For this review, take the finished solid that the model builds, in its own axes (mm). Round coordinates to 2 decimals unless told otherwise and drop trailing zeros. Order: outer loops, then holes, each group sorted by start corner. A loop starts at its lowest first (then second) coordinate and runs counter-clockwise, first axis right, second up. Notation, with made-up numbers: (-34.5, 44) - (-2.5, 44) arc R9 cw to (-2.5, 50) - close; hole circle Ø5 at (-12.5, 11). An arc over 180 degrees is marked (long way). One line per item, written item: value.
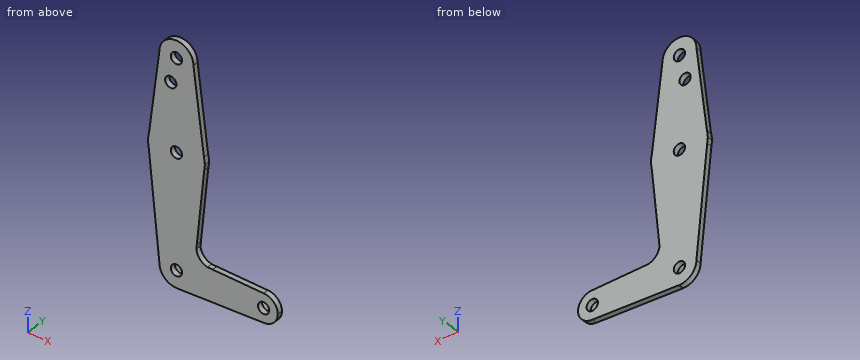
```python
from build123d import *

# Parameters (mm, degrees)
F0_R     = 3.175
F1_DEPTH = 3.048


with BuildPart() as f1:
    # F0 (on Front) → F1 (new body)
    with BuildSketch(Plane.XZ):
        with BuildLine():
            ThreePointArc((-9.525, 66.5221907973), (0, 56.9971907973), (9.525, 66.5221907973))
            ThreePointArc((9.525, 66.5221907973), (0, 76.0471907973), (-9.525, 66.5221907973))
        make_face()
        with Locations((0, 66.5221907973)):
            Circle(F0_R, mode=Mode.SUBTRACT)
        with BuildLine():
            Line((15.3865384615, 19.629883105), (9.525, 66.5221907973))
            ThreePointArc((9.525, 66.5221907973), (0, 56.9971907973), (-9.525, 66.5221907973))
            Line((-9.525, 66.5221907973), (-15.3865384615, 19.629883105))
            ThreePointArc((-15.3865384615, 19.629883105), (0, 31.5971907973), (15.3865384615, 19.629883105))
        make_face()
        with Locations((-3.175, 52.341658622)):
            Circle(F0_R, mode=Mode.SUBTRACT)
        with BuildLine():
            Line((15.875, 15.7221907973), (15.3865384615, 19.629883105))
            ThreePointArc((15.3865384615, 19.629883105), (0, 31.5971907973), (-15.3865384615, 19.629883105))
            Line((-15.3865384615, 19.629883105), (-15.875, 15.7221907973))
            Line((-15.875, 15.7221907973), (-15.5606435644, 12.5786264409))
            ThreePointArc((-15.5606435644, 12.5786264409), (0, -0.1528092027), (15.5606435644, 12.5786264409))
            Line((15.5606435644, 12.5786264409), (15.875, 15.7221907973))
        make_face()
        with Locations((0, 15.7221907973)):
            Circle(F0_R, mode=Mode.SUBTRACT)
        with BuildLine():
            ThreePointArc((15.875, 15.7221907973), (15.7524112928, 17.6912422089), (15.3865384615, 19.629883105))
            Line((15.3865384615, 19.629883105), (15.875, 15.7221907973))
        make_face()
        with BuildLine():
            Line((-15.875, 15.7221907973), (-15.3865384615, 19.629883105))
            ThreePointArc((-15.3865384615, 19.629883105), (-15.7524112928, 17.6912422089), (-15.875, 15.7221907973))
        make_face()
        with BuildLine():
            ThreePointArc((15.5606435644, 12.5786264409), (15.7962153946, 14.1425692579), (15.875, 15.7221907973))
            Line((15.875, 15.7221907973), (15.5606435644, 12.5786264409))
        make_face()
        with BuildLine():
            Line((-15.5606435644, 12.5786264409), (-15.875, 15.7221907973))
            ThreePointArc((-15.875, 15.7221907973), (-15.7962153946, 14.1425692579), (-15.5606435644, 12.5786264409))
        make_face()
        with BuildLine():
            Line((11.4104326497, -28.9234827055), (15.5606435644, 12.5786264409))
            ThreePointArc((15.5606435644, 12.5786264409), (0, -0.1528092027), (-15.5606435644, 12.5786264409))
            Line((-15.5606435644, 12.5786264409), (-9.525, -47.7778092027))
            ThreePointArc((-9.525, -47.7778092027), (-6.7351920908, -41.0426171119), (0, -38.2528092027))
            ThreePointArc((0, -38.2528092027), (0.309842749, -38.2578500394), (0.6193575471, -38.272967214))
            Line((0.6193575471, -38.272967214), (10.4435098772, -38.5927104307))
            Line((10.4435098772, -38.5927104307), (11.1406480746, -31.6213284562))
            ThreePointArc((11.1406480746, -31.6213284562), (11.1596842937, -30.260819974), (11.4104326497, -28.9234827055))
        make_face()
        with BuildLine():
            Line((11.1406480746, -31.6213284562), (11.4104326497, -28.9234827055))
            ThreePointArc((11.4104326497, -28.9234827055), (11.1596842937, -30.260819974), (11.1406480746, -31.6213284562))
        make_face()
        with BuildLine():
            ThreePointArc((0, -38.2528092027), (-6.7351920908, -41.0426171119), (-9.525, -47.7778092027))
            ThreePointArc((-9.525, -47.7778092027), (-6.7351920908, -54.5130012935), (0, -57.3028092027))
            Line((0, -57.3028092027), (0.6193575471, -57.2826511913))
            ThreePointArc((0.6193575471, -57.2826511913), (6.9507195899, -54.2903449747), (9.525, -47.7778092027))
            ThreePointArc((9.525, -47.7778092027), (6.9507195899, -41.2652734306), (0.6193575471, -38.272967214))
            Line((0.6193575471, -38.272967214), (0, -38.2528092027))
        make_face()
        with Locations((0, -47.7778092027)):
            Circle(F0_R, mode=Mode.SUBTRACT)
        with BuildLine():
            ThreePointArc((17.370144363, -38.8181491572), (13.0593477477, -36.2550264457), (11.1406480746, -31.6213284562))
            Line((11.1406480746, -31.6213284562), (10.4435098772, -38.5927104307))
            Line((10.4435098772, -38.5927104307), (17.370144363, -38.8181491572))
        make_face()
        with BuildLine():
            Line((0.6193575471, -57.2826511913), (0, -57.3028092027))
            ThreePointArc((0, -57.3028092027), (0.309842749, -57.297768366), (0.6193575471, -57.2826511913))
        make_face()
        with BuildLine():
            Line((17.370144363, -38.8181491572), (10.4435098772, -38.5927104307))
            Line((10.4435098772, -38.5927104307), (9.525, -47.7778092027))
            ThreePointArc((9.525, -47.7778092027), (6.9507195899, -54.2903449747), (0.6193575471, -57.2826511913))
            Line((0.6193575471, -57.2826511913), (48.7761460245, -55.7153092027))
            ThreePointArc((48.7761460245, -55.7153092027), (40.8386460245, -47.7778092027), (48.7761460245, -39.8403092027))
            Line((48.7761460245, -39.8403092027), (20.2621190411, -38.9122732358))
            ThreePointArc((20.2621190411, -38.9122732358), (18.8118135488, -38.9978870226), (17.370144363, -38.8181491572))
        make_face()
        with BuildLine():
            Line((20.2621190411, -38.9122732358), (17.370144363, -38.8181491572))
            ThreePointArc((17.370144363, -38.8181491572), (18.8118135488, -38.9978870226), (20.2621190411, -38.9122732358))
        make_face()
        with BuildLine():
            ThreePointArc((48.7761460245, -39.8403092027), (40.8386460245, -47.7778092027), (48.7761460245, -55.7153092027))
            ThreePointArc((48.7761460245, -55.7153092027), (54.3888061001, -53.3904692783), (56.7136460245, -47.7778092027))
            ThreePointArc((56.7136460245, -47.7778092027), (54.3888061001, -42.165149127), (48.7761460245, -39.8403092027))
        make_face()
        with Locations((48.7761460245, -47.7778092027)):
            Circle(F0_R, mode=Mode.SUBTRACT)
        with BuildLine():
            Line((9.525, -47.7778092027), (10.4435098772, -38.5927104307))
            Line((10.4435098772, -38.5927104307), (0.6193575471, -38.272967214))
            ThreePointArc((0.6193575471, -38.272967214), (6.9507195899, -41.2652734306), (9.525, -47.7778092027))
        make_face()
    extrude(amount=F1_DEPTH)


solid = f1.part
```
Item 1: Wall thickness on line 1 (Z direction, x = 46, y = -2.8); line 2 (X direction, y = -2.7, z = 17.5); line 3 (X direction, y = -1.45, z = 11): over which ranges is each line inside the solid? List them lowest first.
Returned:
line 1: -55.81 to -49.32, -46.24 to -39.75
line 2: -15.78 to -2.63, 2.63 to 15.78
line 3: -15.4 to 15.4
Item 2: Take a section at B-B (x = -1.5). Write out the cut boundary in (y, z), plus the area to 3 significant figures.
Returned:
outline: (-3.05, -57.18) - (0, -57.18) - (0, -50.58) - (-3.05, -50.58) - close; (-3.05, -44.98) - (0, -44.98) - (0, 12.92) - (-3.05, 12.92) - close; (-3.05, 18.52) - (0, 18.52) - (0, 49.64) - (-3.05, 49.64) - close; (-3.05, 55.04) - (0, 55.04) - (0, 63.72) - (-3.05, 63.72) - close; (-3.05, 69.32) - (0, 69.32) - (0, 75.93) - (-3.05, 75.93) - close
area: 338 mm^2
Item 3: Take a section at A-A (z = 14). Write out the cut boundary in (x, y).
Returned:
outline: (-15.78, -3.05) - (-2.67, -3.05) - (-2.67, 0) - (-15.78, 0) - close; (2.67, -3.05) - (15.78, -3.05) - (15.78, 0) - (2.67, 0) - close
Item 4: For P1, Ø1, axis at y = -2, z = -22.5, coming from the -X side; P2, Ø1, axis at x = 5, y = -2.5, coming from the +Z side; P3, Ø1.5, axis at x = 11, y = -1.5, coming from the -Z side, all flat-tipped, find the tip position at first contact; note any pin that passes through.
Returned:
P1: x = -12.1
P2: z = 74.92
P3: z = -56.97
Item 5: Take a section at D-D (x = 22.5). Write out the cut boundary in (y, z).
Returned:
outline: (-3.05, -56.57) - (0, -56.57) - (0, -38.99) - (-3.05, -38.99) - close
